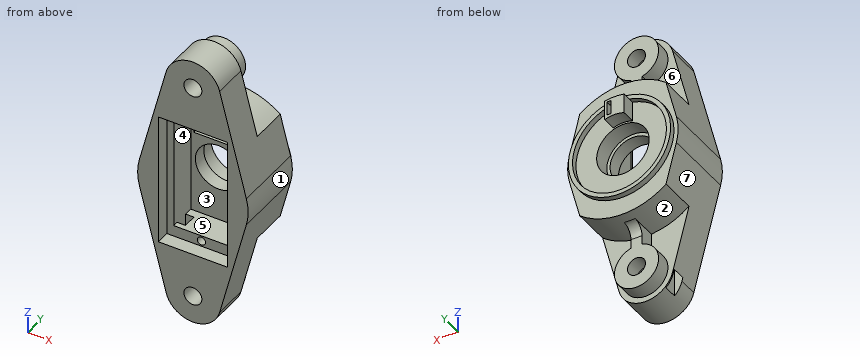
Autodesk Inventor part; units mm, degrees
ref_plane "YZ Plane" through (0, 0, 0) normal (1, 0, 0) x (0, 1, 0)
ref_plane "XZ Plane" through (0, 0, 0) normal (0, 1, 0) x (-1, 0, 0)
ref_plane "XY Plane" through (0, 0, 0) normal (0, 0, 1) x (1, 0, 0)
sketch "Sketch1" plane through (0, 0, 0) normal (1, 0, 0) x (0, 1, 0)
  line L0 (121, 3) -> (1, 3)
  line L1 (1, 3) -> (1, -3)
  line L2 (1, -3) -> (121, -3)
  line L3 (121, -3) -> (121, 3)
  line L4 (121, 3) -> (1, -3) construction
  line L5 (1, 3) -> (121, -3) construction
  line L6 (10, 8.35) -> (0, 8.35)
  line L7 (0, 8.35) -> (0, 20)
  line L8 (10, 8.35) -> (10, 9.5)
  line L9 (10, 9.5) -> (16, 9.5)
  line L10 (16, 9.5) -> (16, 17)
  line L11 (16, 17) -> (18, 17)
  line L12 (18, 17) -> (18, 18.5)
  line L13 (18, 18.5) -> (16, 18.5)
  line L14 (16, 18.5) -> (16, 20)
  line L15 (16, 20) -> (0, 20)
  line L16 (-36.2, 0) -> (147.2, 0)
  line L17 (16, 20) -> (31, 20)
  line L18 (18, 17) -> (31, 17)
  line L19 (75, 9.45) -> (69, 9.45)
  line L20 (69, 9.45) -> (69, 8.35)
  line L21 (69, 8.35) -> (66, 8.35)
  line L22 (75, 9.45) -> (75, 12.45)
  arc A0 (75, 12.45) -> (31, 20) centre (31, -111.9869) ccw
  arc A1 (59.1084, 13.9001) -> (31, 17) centre (31, -111.9869) ccw
  arc A2 (66, 8.35) -> (59.1084, 13.9001) centre (56.9292, 4.1404) ccw
  line L23 (0, 20) -> (-10, 20)
  line L24 (-10, 20) -> (-10, 8.35)
  line L25 (-10, 8.35) -> (0, 8.35)
  line L26 (0, 8.35) -> (0, 20)
  point P0 (0, 0)
  point P1 (61, 0)
  point P2 (61, 0)
  dimension "d0" = 120
  dimension "d1" = 6
  dimension "d5" = 8.35
  dimension "d6" = 9.5
  dimension "d7" = 1.5
  dimension "d8" = 1.5
  dimension "d9" = 20
  dimension "d10" = 6
  dimension "d11" = 2
  dimension "d13" = 10
  dimension "d14" = 1
  dimension "d15" = 6
  dimension "d16" = 3
  dimension "d17" = 9.45
  dimension "d18" = 3
  dimension "d19" = 8.35
  dimension "d20" = 15
  dimension "d21" = 7.5
  dimension "d22" = 75
  dimension "d23" = 10
  dimension "d42" = 10
  dimension "d43" = 8.35
revolve "Revolution1" add sketch "Sketch1" angle 360 about axis through (0, -10, 0) along (0, 1, 0) contours L6 L7 L15 L14 L13 L12 L11 L10 L9 L8 | L25 L24 L23 L7
sketch "Sketch2" plane through (0, 0, 0) normal (0, 1, 0) x (-1, 0, 0)
  circle A0 centre (0, 0) radius 20
  circle A1 centre (0, 40) radius 3.25
  line L0 (28, 0) -> (-28, 0)
  line L1 (19.3649, 5) -> (9.6825, 42.5)
  line L2 (-19.3649, 5) -> (-9.6825, 42.5)
  arc A2 (9.6825, 42.5) -> (-9.6825, 42.5) centre (0, 40) ccw
  circle A3 centre (0, 40) radius 8
  arc A4 (15.6149, 19.5237) -> (-15.6149, 19.5237) centre (0, 0) ccw
  line L3 (2, 32.254) -> (2, 24.9199)
  line L4 (-2, 32.254) -> (-2, 24.9199)
  dimension "d25" = 6.5
  dimension "d28" = 10
  dimension "d29" = 16
  dimension "d30" = 5
  dimension "d31" = 40
  dimension "d34" = 4
extrude "Extrusion1" add sketch "Sketch2" along normal blind 2.5 and the other way blind 10 contours A0 L2 A4 L1 | A4 L3 A3 L4 L2 A2 L1 | A4 L4 A3 L3 | A3 | A1
extrude "Extrusion2" add sketch "Sketch2" along normal up to surface (26 mm away) from surface at -10 contours A0 L2 A4 L1
extrude "Extrusion3" add sketch "Sketch2" along normal blind 8 contours A4 L4 A3 L3 | A3
fillet "Fillet1" radius 4 1 edges at (0, 8, 25)
mirror "Mirror1" about plane through (0, 0, 0) normal (0, 0, 1) of "Extrusion2", "Extrusion3", "Fillet1", "Extrusion1"
sketch "Sketch3" plane through (0, -10, 0) normal (0, -1, 0) x (0, 0, 1)
  line L0 (5, -19.3649) -> (42.5, -9.6825)
  circle A0 centre (0, 0) radius 8.35
  arc A1 (-5, -19.3649) -> (5, -19.3649) centre (0, 0) ccw
  line L1 (5, -19.3649) -> (42.5, -9.6825)
  line L2 (42.5, 9.6825) -> (5, 19.3649)
  arc A2 (5, 19.3649) -> (-5, 19.3649) centre (0, 0) ccw
  line L3 (-42.5, 9.6825) -> (-5, 19.3649)
  line L4 (-5, -19.3649) -> (-42.5, -9.6825)
  circle A3 centre (0, 0) radius 8.35
  arc A4 (-5, -19.3649) -> (5, -19.3649) centre (0, 0) ccw
  line L5 (5, -19.3649) -> (42.5, -9.6825)
  line L6 (42.5, 9.6825) -> (5, 19.3649)
  arc A5 (5, 19.3649) -> (-5, 19.3649) centre (0, 0) ccw
  line L7 (-42.5, 9.6825) -> (-5, 19.3649)
  line L8 (-5, -19.3649) -> (-42.5, -9.6825)
  line L9 (20, 10) -> (-20, 10)
  line L10 (-20, 10) -> (-20, -10)
  line L11 (-20, -10) -> (20, -10)
  line L12 (20, -10) -> (20, 10)
  arc A6 (42.5, -9.6825) -> (42.5, 9.6825) centre (40, 0) ccw
  arc A7 (-42.5, 9.6825) -> (-42.5, -9.6825) centre (-40, 0) ccw
  arc A8 (42.5, -9.6825) -> (42.5, 9.6825) centre (40, 0) ccw
  arc A9 (-42.5, 9.6825) -> (-42.5, -9.6825) centre (-40, 0) ccw
  point P0 (15.6149, 19.5237)
  dimension "d44" = 0
  dimension "d45" = 0
  dimension "d59" = 40
  dimension "d60" = 10
  dimension "d61" = 10
extrude "Extrusion5" cut sketch "Sketch3" against normal blind 15 contours L12 L11 L10 L9
sketch "Sketch4" plane through (0, -10, 0) normal (0, -1, 0) x (0, 0, 1)
  line L0 (-20, -10) -> (-20, 10)
  line L1 (-20, 10) -> (20, 10)
  line L2 (20, 10) -> (20, -10)
  line L3 (20, -10) -> (-20, -10)
  arc A0 (-5, -19.3649) -> (5, -19.3649) centre (0, 0) ccw
  line L4 (5, -19.3649) -> (42.5, -9.6825)
  line L5 (42.5, 9.6825) -> (5, 19.3649)
  arc A1 (5, 19.3649) -> (-5, 19.3649) centre (0, 0) ccw
  line L6 (-42.5, 9.6825) -> (-5, 19.3649)
  line L7 (-5, -19.3649) -> (-42.5, -9.6825)
  line L8 (24, 12.5) -> (-24, 12.5)
  line L9 (-24, 12.5) -> (-24, -12.5)
  line L10 (-24, -12.5) -> (24, -12.5)
  line L11 (24, -12.5) -> (24, 12.5)
  arc A2 (42.5, -9.6825) -> (42.5, 9.6825) centre (40, 0) ccw
  arc A3 (-42.5, 9.6825) -> (-42.5, -9.6825) centre (-40, 0) ccw
  dimension "d51" = 4
  dimension "d52" = 2.5
  dimension "d53" = 4
  dimension "d54" = 2.5
extrude "Extrusion6" cut sketch "Sketch4" against normal blind 5 contours L11 L10 L9 L8
sketch "Sketch6" plane through (0, 16, 0) normal (0, 1, 0) x (1, 0, 0)
  circle A0 centre (0, 0) radius 17
  circle A1 centre (0, 0) radius 9.5
  line L0 (3.5, -16.6358) -> (3.5, -10.1358)
  line L1 (-3.5, -10.1358) -> (-3.5, -16.6358)
  arc A2 (-3.5, -16.6358) -> (3.5, -16.6358) centre (0, 0) ccw
  arc A3 (-3.5, -9.5123) -> (3.5, -9.5123) centre (0, 0) ccw
  line L2 (-3.5, -9.5123) -> (-3.5, -10.1358)
  line L3 (-12.5, 24) -> (-12.5, -24)
  line L4 (3.5, -9.5123) -> (3.5, -10.1358)
  dimension "d69" = 3.5
  dimension "d70" = 3.5
  dimension "d75" = 0
  dimension "d76" = 0
  dimension "d77" = 40.402
extrude "Extrusion7" add sketch "Sketch6" along normal blind 5 contours L1 L2 A3 L4 L0 A0
sketch "Sketch7" plane through (0, 21, 0) normal (0, 1, 0) x (1, 0, 0)
  line L0 (1.2, -16) -> (2.7, -16)
  line L1 (2.7, -16) -> (2.7, -11)
  line L2 (2.7, -11) -> (1.2, -11)
  line L3 (1.2, -11) -> (1.2, -16)
  arc A0 (-3.5, -9.5123) -> (3.5, -9.5123) centre (0, 0) ccw
  dimension "d79" = 11
  dimension "d80" = 5
  dimension "d81" = 1.5
  dimension "d82" = 1.2
extrude "Extrusion8" cut sketch "Sketch7" against normal up to surface (16 mm away)
sketch "Sketch8" plane through (0, 2.5, 0) normal (0, 1, 0) x (1, 0, 0)
  circle A0 centre (0, -40) radius 3.25
  circle A1 centre (0, 40) radius 3.25
  point P0 (0, 0)
extrude "Extrusion9" cut sketch "Sketch8" against normal up to surface (12.5 mm away)
sketch "Sketch9" plane through (-10, 5, -20) normal (0, 0, 1) x (1, 0, 0)
  point P0 (10, -5)
sketch "Sketch10" plane through (-10, 5, -20) normal (0, 0, 1) x (1, 0, 0)
  line L0 (0, -10) -> (0, 0)
  line L1 (0, -8) -> (3, -8)
  line L2 (3, -8) -> (3, -3)
  line L3 (3, -3) -> (0, -3)
  line L4 (0, -3) -> (0, -8)
  line L5 (0, -10) -> (20, -10)
  line L6 (20, -10) -> (20, 0)
  line L7 (20, 0) -> (0, 0)
  line L8 (0, -10) -> (0, 0)
  point P0 (10, -5)
  point P1 (0, -2.5)
  dimension "d87" = 2
  dimension "d88" = 5
  dimension "d89" = 3
extrude "Extrusion10" cut sketch "Sketch10" against normal blind 30 contours L0 L3 L2 L1
sketch "Sketch11" plane through (0, -5, 0) normal (0, -1, 0) x (1, 0, 0)
  line L0 (-10, -20) -> (10, -20)
  line L1 (10, -20) -> (10, 20)
  line L2 (-10, -20) -> (10, -20)
  line L3 (-10, 20) -> (-10, -20)
  line L4 (10, 20) -> (-10, 20)
  line L5 (-12.5, -24) -> (-12.5, 24)
  line L6 (12.5, -24) -> (-12.5, -24)
  line L7 (12.5, 24) -> (12.5, -24)
  line L8 (-12.5, 24) -> (12.5, 24)
  circle A0 centre (0, -22) radius 1.5
  circle A1 centre (0, 22) radius 1.5
  point P0 (0, 0)
  dimension "d92" = 3
  dimension "d93" = 3
  dimension "d94" = 22
  dimension "d95" = 22
  dimension "d96" = 0
  dimension "d97" = 0
extrude "Extrusion11" cut sketch "Sketch11" against normal blind 20 contours A0 | A1
sketch "Sketch12" plane through (-19.3649, -10, -5) normal (-0.9682, 0, -0.25) x (-0.25, 0, 0.9682)
  point P0 (0, 10)
sketch "Sketch14" plane through (0, 5, 0) normal (0, -1, 0) x (1, 0, 0)
  line L0 (2.7, 16) -> (2.7, 11)
  line L1 (1.2, 11) -> (1.2, 16)
  line L2 (2.7, 11) -> (1.2, 11)
  line L3 (1.2, 16) -> (2.7, 16)
  line L4 (-8.8, 19) -> (8.7, 19)
  line L5 (8.7, 19) -> (8.7, 10)
  line L6 (8.7, 10) -> (-8.8, 10)
  line L7 (-8.8, 10) -> (-8.8, 19)
  line L8 (-10, 20) -> (10, 20)
  point P0 (0, 0)
  dimension "d101" = 1
  dimension "d102" = 6
  dimension "d103" = 10
  dimension "d106" = 1
extrude "Extrusion12" cut sketch "Sketch14" against normal blind 8
equation "\"d54\" = d52"
properties part number "Base"
Input: part model. Units: mm. Frame: model coordinates. Face numbers are marked on the shaded views. A direction names the side the tool comes from. Give positions to 0.01 mm unless a question says otherwise; leave off trailing zeros. Write each loop counter-clockwise with the first axis right and the second up, starting at its lowest first coordinate (ties: lowest second). Pieces come first, ordered by that corner, then holes.
Q1. Set-up query: the marked faces 4, 5, 6 and 7. Return all of +Z, -Z, +X, -X, +Y, -Y with unobstructed straight access to the full face (end or side cutting, diameter ignored); none if empty.
Q2. Section C-C, the plane z = -22. Output: boundary loops of the cut face in (x, y).
Q3. Material intervals for probe 1 along Z at (x, y) = (0, 1); probe 2 along Z at (x, y) = (-6, 11); probe 3 along X at (y, z) = (20, 13.5), sorted ascending.
Q4. Section B-B, the plane y = 0.5. Output: boundary loops of the cut face in (x, z), plus the area to 3 significant figures.
Q5. First-contact query: P1, Ø2.5, axis at x = 0, z = 22, coming from the +Y side; P2, Ø2, axis at y = 8, z = 28.5, coming from the -X side; P3, Ø1.2, axis at x = 1.5, y = 17, coming from the +Z side. Flat tips, straight axial feed; report the tip coordinate or a pass-through.
Q6. Section A-A, the plane z = 40. Output: boundary loops of the cut face in (x, y), plus the area to 3 significant figures.
Q7. Pull-direction query (X, two-part tool) for the marked faces 1, 2 and 3; classes: pulls with the +X half, pulls with the -X half, needs draft (parallel to the pull), parting line crosses it, or undercut.
Q8. Section D-D, the plane x = 0. State how many separate pieces and enclosed holes the cut face has, plus the area to 3 significant figures.
Filled in:
1. face 4: none
1. face 5: -Y
1. face 6: +Y
1. face 7: -Z, -X, +Y, -Y
2. outline: (-14.98, -10) - (-12.5, -10) - (-12.5, -5) - (-1.5, -5) - (-1.5, 15) - (1.5, 15) - (1.5, -5) - (12.5, -5) - (12.5, -10) - (14.98, -10) - (14.98, 2.5) - (11.87, 2.5) - (11.87, 16) - (-11.87, 16) - (-11.87, 2.5) - (-14.98, 2.5) - close; hole (-10, -3) - (-7, -3) - (-7, 2) - (-10, 2) - close
3. probe 1: z = -50 to -43.25, -36.75 to -23.5, -20.5 to -20, 20 to 20.5, 23.5 to 36.75, 43.25 to 50
3. probe 2: z = -24.27 to -7.37, 7.37 to 10, 19 to 24.27
3. probe 3: x = -3.5 to 1.2, 2.7 to 3.5
4. outline: (-19.36, -5) - (-10, -41.27) - (-10, 20) - (10, 20) - (10, -20) - (-7, -20) - (-7, -47.14) arc R10 ccw to (9.68, -42.5) - (19.36, -5) arc R20 ccw to (19.36, 5) - (9.68, 42.5) arc R10 ccw to (-9.68, 42.5) - (-19.36, 5) arc R20 ccw to start; hole circle Ø6.5 at (0, -40); hole circle Ø6.5 at (0, 40); hole circle Ø3 at (0, -22); hole circle Ø3 at (0, 22)
4. area: 1,830 mm2
5. P1: stops at y = 16
5. P2: stops at x = -2
5. P3: stops at z = 18.48
6. outline: (-10.33, -10) - (-3.25, -10) - (-3.25, 8) - (-8, 8) - (-8, 2.5) - (-10.33, 2.5) - close; (3.25, -10) - (10.33, -10) - (10.33, 2.5) - (8, 2.5) - (8, 8) - (3.25, 8) - close
6. area: 229 mm2
7. face 1: pulls with the +X half
7. face 2: parting line crosses it
7. face 3: undercut
8. separate pieces: 4
8. enclosed holes: 0
8. area: 962 mm2
